from build123d import *

# Parameters (mm, degrees)
SKETCH1_W           = 28.74
SKETCH1_H           = 33.5
BOSS_EXTRUDE1_DEPTH = 3.5


with BuildPart() as part:
    # Sketch1 → Boss-Extrude1 (new body)
    with BuildSketch(Plane(origin=(0, 0, 0), x_dir=(1, 0, 0), z_dir=(0, 1, 0))):
        Rectangle(SKETCH1_W, SKETCH1_H)
    extrude(amount=BOSS_EXTRUDE1_DEPTH)

    # Sketch4 → Revolve1 (revolve)
    with BuildSketch(Plane(origin=(0, 0, 0), x_dir=(0, 0, -1), z_dir=(1, 0, 0))):
        with BuildLine():
            Line((0, 0), (-11, 0))
            Line((-11, 0), (-11, 3.4))
            ThreePointArc((-11, 3.4), (-7.813771351, 11.243059943), (0, 14.500454536))
            Line((0, 14.500454536), (0, 0))
        make_face()
    revolve(axis=Axis((0, 14.500454536, 0), (0, -1, 0)))


solid = part.part
The listing builds one solid part. Answer for the finished solid, in the listing's coordinates (mm). A direction names the side the tool comes from. Round coordinates to 2 decimals unless told otherwise and drop trailing zeros. Order: outer loops, then holes, each group sorted by start corner. A loop starts at its lowest first (then second) coordinate and runs counter-clockwise, first axis right, second up. Notation, with made-up numbers: (-8.5, 4.5) -> (44.5, 4.5) arc R13 cw to (44.5, 23.5) -> close; hole circle Ø7 at (-36, -25.75). An arc over 180 degrees is marked (long way). One line per item, written item: value.
Item 1: Given P1, Ø3, axis at y = 7, z = 7, coming from the +X side; P2, Ø2, axis at x = -3.5, y = 6, coming from the +Z side; P3, Ø1.5, axis at y = 6, z = -10.5, coming from the -X side, each flat-ended and moving along its own axis, determine where each tip first touches the part or whether it passes through.
Taken from the geometry:
P1: stops at x = 9
P2: stops at z = 10.49
P3: stops at x = -4.49
Item 2: Find section A-A, the plane x = 1.5. Give the vertices of the cut face in (y, z), then the cut area to 3 significant figures.
Taken from the geometry:
outline: (0, -16.75) -> (3.5, -16.75) -> (3.5, -10.9) arc R10.9 ccw to (3.5, 10.9) -> (3.5, 16.75) -> (0, 16.75) -> close
area: 304 mm2
Item 3: For faces 1 (the flat face through (-14.37, 2, 0)), 2 (the flat face through (-0.2, 3.5, -11.4)), determine the directions among +Z, -Z, +X, -X, +Y, -Y from which every point of the face is accessible in a straight line to the end or side of a thin tool.
Taken from the geometry:
face 1: +Z, -Z, -X, +Y, -Y
face 2: +Y
Item 4: Straight lines are drawn through the part: L1, parallel to Y at x = -8.25, z = 11; L2, parallel to X at y = 9.75, z = -6; L3, parallel to Z at x = -4, y = 9. For each, find the intervals that lie inside material, in ascending order.
Taken from the geometry:
L1: y = 0 to 3.5
L2: x = -6.78 to 6.78
L3: z = -8.65 to 8.65
Item 5: Find section B-B, the plane z = 13. Give the vertices of the cut face in (x, y), then the cut area to 3 significant figures.
Taken from the geometry:
outline: (-14.37, 0) -> (14.37, 0) -> (14.37, 3.5) -> (-14.37, 3.5) -> close
area: 101 mm2
Item 6: Find section D-D, the plane z = 5. Give the vertices of the cut face in (x, y).
Taken from the geometry:
outline: (-14.37, 0) -> (14.37, 0) -> (14.37, 3.5) -> (9.8, 3.5) arc R9.8 ccw to (-9.8, 3.5) -> (-14.37, 3.5) -> close
Item 7: Find section C-C, the plane y = 11.75. Give the vertices of the cut face in (x, z).
Taken from the geometry:
outline: circle Ø14.55 at (0, 0)
